Autodesk Inventor part; units mm, degrees
ref_plane "YZ Plane" through (0, 0, 0) normal (1, 0, 0) x (0, 1, 0)
ref_plane "XZ Plane" through (0, 0, 0) normal (0, 1, 0) x (-1, 0, 0)
ref_plane "XY Plane" through (0, 0, 0) normal (0, 0, 1) x (1, 0, 0)
sketch "Sketch1" plane through (0, 0, 0) normal (0, 1, 0) x (-1, 0, 0)
  line L0 (0, -232.2291) -> (0, -361.7009)
  line L1 (0, -361.7009) -> (63.5, -361.7009)
  line L2 (63.5, -361.7009) -> (63.5, -95.0009)
  line L3 (63.5, -95.0009) -> (135.342, -23.1589)
  line L4 (135.342, -23.1589) -> (503.642, -23.1589)
  line L5 (503.642, -23.1589) -> (503.642, 40.3411)
  line L6 (503.642, 40.3411) -> (59.142, 40.3411)
  line L7 (59.142, 40.3411) -> (0, -18.8009)
  line L8 (0, -18.8009) -> (0, -232.2291)
  line L9 (99.421, -59.0799) -> (29.571, 10.7701) construction
  circle A0 centre (86.8487, -46.5075) radius 2.54
  circle A1 centre (50.9276, -10.5865) radius 1.7463
  point P0 (0, 0)
  dimension "d0" = 63.5
  dimension "d2" = 63.5
  dimension "d3" = 101.6
  dimension "d4" = 266.7
  dimension "d5" = 368.3
  dimension "d6" = 342.9
  dimension "d7" = 444.5
  dimension "d10" = 5.08
  dimension "d11" = 17.78
  dimension "d12" = 3.4925
  dimension "d13" = 68.58
extrude "Extrusion1" add sketch "Sketch1" along normal blind 3.4925
properties part number "OptiTrack_Calibrator"
Can you work these out from the model? Positions are in its coordinate system, mm. Round coordinates to 2 decimals unless told otherwise and drop trailing zeros. Loops run counter-clockwise (first coordinate to the right, second up) from the corner with the lowest first, then second, coordinate; pieces in that order, holes last.
Item 1: Suppose I cut it at C-C, the plane z = -275. Write out the boundary of the cut face in (x, y).
Item 2: Will these pins go through, and if not, where does the flat tip stop? pin 1 Ø1 at (y, z) = (1, -193) entering from -X; pin 2 Ø4.5 at (x, z) = (-86.85, -46.51) entering from +Y; pin 3 Ø1 at (x, y) = (-296, 1) entering from -Z.
Item 3: Suppose I cut it at B-B, the plane x = -238. Write out the boundary of the cut face in (y, z), then the cut area to 3 significant figures.
Item 4: Please list where these lines run through material, in increasing order: L1, parallel to Z at x = -447, y = 1.6; L2, parallel to X at y = 1.4, z = -201; L3, parallel to Z at x = -97.5, y = 0.2.
Item 5: Suppose I cut it at A-A, the plane y = 2.9. Write out the boundary of the cut face in (x, z), then the cut area to 3 significant figures.
Reported:
1. outline: (-63.5, 0) - (0, 0) - (0, 3.49) - (-63.5, 3.49) - close
2. pin 1: stops at x = -63.5
2. pin 2: passes through
2. pin 3: stops at z = -23.16
3. outline: (0, -23.16) - (3.49, -23.16) - (3.49, 40.34) - (0, 40.34) - close
3. area: 222 mm2
4. L1: z = -23.16 to 40.34
4. L2: x = -63.5 to 0
4. L3: z = -61 to 40.34
5. outline: (-503.64, -23.16) - (-135.34, -23.16) - (-63.5, -95) - (-63.5, -361.7) - (0, -361.7) - (0, -18.8) - (-59.14, 40.34) - (-503.64, 40.34) - close; hole circle Ø5.08 at (-86.85, -46.51); hole circle Ø3.49 at (-50.93, -10.59)
5. area: 54,300 mm2
